Can you work these out from the drawing? Everything is in mm from the part's minimum corner. Coordinates: 2 decimals unless noted, no trailing zeros. Order: outer loops, then holes, each group sorted by start corner. A loop starts at its lowest first (then second) coordinate and runs counter-clockwise, first axis right, second up. Notation, with made-up numbers: M 76.5,23 L 98.5,23 A20 ccw 98.5,46 Z; hole C -21,40.25 d11. An arc over 180 degrees is marked long. Answer as a JSON object with one key per item and string values.
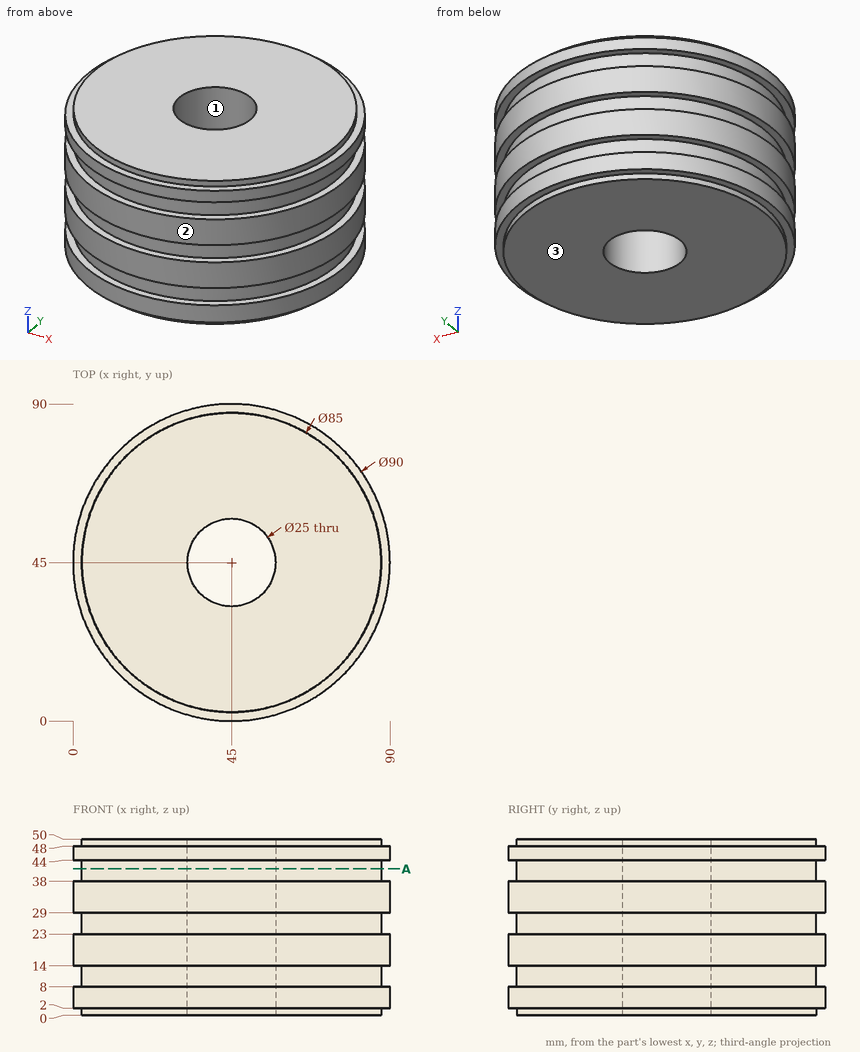
Item 1: I want a section at A-A, the plane z = 41.5. Write out the boundary of the cut face in (x, y).
Answers follow:
{"outline": "C 45,45 d85; hole C 45,45 d25"}
Item 2: If we mould it in two halves opening along Y, with no side actions, what happens to the marked faces 1, 2 and 3? For each: pulls with the +Y half, pulls with the -Y half, needs draft (parallel to the pull), parting line crosses it, or undercut.
Answers follow:
{"face 1": "undercut", "face 2": "parting line crosses it", "face 3": "needs draft"}
Item 3: Please list where these lines run through material, in increasing order: line 1 (Y direction, x = 45, z = 20.5); line 2 (X direction, y = 35, z = 32); line 3 (Y direction, x = 43, z = 21).
Answers follow:
{"line 1": "y = 0 to 32.5, 57.5 to 90", "line 2": "x = 1.13 to 37.5, 52.5 to 88.87", "line 3": "y = 0.04 to 32.66, 57.34 to 89.96"}
Item 4: I'm going to push flat-ended pins straight in: pin 1 (12 mm diameter, centred on y = 27.5, z = 8.5, fed in from -X); pin 2 (6 mm diameter, centred on y = 14.5, z = 37.5, fed in from -X); pin 3 (5 mm diameter, centred on x = 16.5, z = 32, fed in from +Y). Where does each tip first touch, or does it pass through?
Answers follow:
{"pin 1": "stops at x = 1.5", "pin 2": "stops at x = 9.38", "pin 3": "stops at y = 81.73"}
